```python
from build123d import *

# Parameters (mm, degrees)
ESQUISSE1_W              = 200
ESQUISSE1_H              = 140
BOSS_EXTRU_1_DEPTH       = 6
ESQUISSE8_W              = 31
ESQUISSE8_H              = 60
ESQUISSE8_W_2            = 10
ENL_V_MAT_EXTRU_2_DEPTH  = 6
ESQUISSE9_W              = 20
ESQUISSE9_H              = 6
ENL_V_MAT_EXTRU_3_DEPTH  = 6
ESQUISSE10_W             = 6
ESQUISSE10_H             = 20
ENL_V_MAT_EXTRU_4_DEPTH  = 6
ESQUISSE14_W             = 30
ESQUISSE14_H             = 6
ENL_V_MAT_EXTRU_7_DEPTH  = 6
ESQUISSE15_R             = 10.5
ENL_V_MAT_EXTRU_8_DEPTH  = 6
ESQUISSE19_R             = 2
ENL_V_MAT_EXTRU_11_DEPTH = 245.204832057
ESQUISSE20_R             = 1.5
ENL_V_MAT_EXTRU_12_DEPTH = 245.204832057
ESQUISSE21_R             = 1.5
ESQUISSE21_W             = 20
ESQUISSE21_H             = 6
ENL_V_MAT_EXTRU_13_DEPTH = 10
ESQUISSE23_R             = 1.65
ENL_V_MAT_EXTRU_15_DEPTH = 6
ESQUISSE16_R             = 1.5
ENL_V_MAT_EXTRU_9_DEPTH  = 6
ESQUISSE28_W             = 6
ESQUISSE28_H             = 20
ENL_V_MAT_EXTRU_17_DEPTH = 245.204832057
ESQUISSE29_R             = 1.5
ENL_V_MAT_EXTRU_18_DEPTH = 245.204832057
ESQUISSE35_R             = 1.5
ENL_V_MAT_EXTRU_21_DEPTH = 6
CONG_1_R                 = 1


with BuildPart() as part:
    # Esquisse1 → Boss.-Extru.1 (new body)
    with BuildSketch(Plane.XY):
        with Locations((100, -70)):
            Rectangle(ESQUISSE1_W, ESQUISSE1_H)
    extrude(amount=BOSS_EXTRU_1_DEPTH)

    # Esquisse8 → Enl_v. mat.-Extru.2 (cut)
    with BuildSketch(Plane(origin=(0, 0, 0), x_dir=(-1, 0, 0), z_dir=(0, 0, -1))):
        with Locations((-146, -42)):
            Rectangle(ESQUISSE8_W, ESQUISSE8_H)
        with Locations((-186, -42)):
            Rectangle(ESQUISSE8_W_2, ESQUISSE8_H)
        with Locations((-14, -42)):
            Rectangle(ESQUISSE8_W_2, ESQUISSE8_H)
        with Locations((-54, -42)):
            Rectangle(ESQUISSE8_W, ESQUISSE8_H)
    extrude(amount=-ENL_V_MAT_EXTRU_2_DEPTH, mode=Mode.SUBTRACT)

    # Esquisse9 → Enl_v. mat.-Extru.3 (cut)
    with BuildSketch(Plane(origin=(0, 0, 0), x_dir=(-1, 0, 0), z_dir=(0, 0, -1))):
        with Locations((-150, -3)):
            Rectangle(ESQUISSE9_W, ESQUISSE9_H)
        with Locations((-50, -3)):
            Rectangle(ESQUISSE9_W, ESQUISSE9_H)
    extrude(amount=-ENL_V_MAT_EXTRU_3_DEPTH, mode=Mode.SUBTRACT)

    # Esquisse10 → Enl_v. mat.-Extru.4 (cut)
    with BuildSketch(Plane(origin=(0, 0, 0), x_dir=(-1, 0, 0), z_dir=(0, 0, -1))):
        with Locations((-197, -100)):
            Rectangle(ESQUISSE10_W, ESQUISSE10_H)
        with Locations((-3, -100)):
            Rectangle(ESQUISSE10_W, ESQUISSE10_H)
    extrude(amount=-ENL_V_MAT_EXTRU_4_DEPTH, mode=Mode.SUBTRACT)

    # Esquisse14 → Enl_v. mat.-Extru.7 (cut)
    with BuildSketch(Plane.XY.offset(6)):
        with Locations((100, -25)):
            Rectangle(ESQUISSE14_W, ESQUISSE14_H)
    extrude(amount=-ENL_V_MAT_EXTRU_7_DEPTH, mode=Mode.SUBTRACT)

    # Esquisse15 → Enl_v. mat.-Extru.8 (cut)
    with BuildSketch(Plane.XY.offset(6)):
        with Locations((195, -135)):
            Circle(ESQUISSE15_R)
        with Locations((5, -135)):
            Circle(ESQUISSE15_R)
    extrude(amount=-ENL_V_MAT_EXTRU_8_DEPTH, mode=Mode.SUBTRACT)

    # Esquisse19 → Enl_v. mat.-Extru.11 (cut, through all)
    with BuildSketch(Plane(origin=(0, 0, 0), x_dir=(-1, 0, 0), z_dir=(0, 0, -1))):
        with Locations((-28.75, -67)):
            Circle(ESQUISSE19_R)
        with Locations((-28.75, -17)):
            Circle(ESQUISSE19_R)
        with Locations(Location((-171.25, -17, 0), (0, 0, 180))):
            Circle(ESQUISSE19_R)
        with Locations(Location((-171.25, -67, 0), (0, 0, 180))):
            Circle(ESQUISSE19_R)
    extrude(amount=-ENL_V_MAT_EXTRU_11_DEPTH, mode=Mode.SUBTRACT)

    # Esquisse20 → Enl_v. mat.-Extru.12 (cut, through all)
    with BuildSketch(Plane.XY.offset(6)):
        with Locations((19.495689014, -120.504310986)):
            Circle(ESQUISSE20_R)
        with Locations((19.212846302, -105.506977889)):
            Circle(ESQUISSE20_R)
        with Locations(Location((180.787153698, -105.506977889, 0), (0, 0, 180))):
            Circle(ESQUISSE20_R)
        with Locations((30, -117.5)):
            Circle(ESQUISSE20_R)
        with Locations((30, -92.5)):
            Circle(ESQUISSE20_R)
        with Locations(Location((180.504310986, -120.504310986, 0), (0, 0, 180))):
            Circle(ESQUISSE20_R)
        with Locations(Location((170, -92.5, 0), (0, 0, 180))):
            Circle(ESQUISSE20_R)
        with Locations(Location((170, -117.5, 0), (0, 0, 180))):
            Circle(ESQUISSE20_R)
        with Locations((76.5, -25)):
            Circle(ESQUISSE20_R)
        with Locations((123.5, -25)):
            Circle(ESQUISSE20_R)
    extrude(amount=-ENL_V_MAT_EXTRU_12_DEPTH, mode=Mode.SUBTRACT)

    # Esquisse21 → Enl_v. mat.-Extru.13 (cut)
    with BuildSketch(Plane(origin=(0, 0, 0), x_dir=(-1, 0, 0), z_dir=(0, 0, -1))):
        with Locations((-85, -71)):
            Circle(ESQUISSE21_R)
        with Locations((-115, -71)):
            Circle(ESQUISSE21_R)
        with Locations((-100, -71)):
            Rectangle(ESQUISSE21_W, ESQUISSE21_H)
    extrude(amount=-ENL_V_MAT_EXTRU_13_DEPTH, mode=Mode.SUBTRACT)

    # Esquisse23 → Enl_v. mat.-Extru.15 (cut)
    with BuildSketch(Plane(origin=(0, 0, 0), x_dir=(-1, 0, 0), z_dir=(0, 0, -1))):
        with Locations(Location((-4.2, -3.5, 0), (0, 0, 180))):
            Circle(ESQUISSE23_R)
        with Locations((-195.8, -3.5)):
            Circle(ESQUISSE23_R)
    extrude(amount=-ENL_V_MAT_EXTRU_15_DEPTH, mode=Mode.SUBTRACT)

    # Esquisse16 → Enl_v. mat.-Extru.9 (cut)
    with BuildSketch(Plane(origin=(0, 0, 0), x_dir=(-1, 0, 0), z_dir=(0, 0, -1))):
        with Locations((-3, -83)):
            Circle(ESQUISSE16_R)
        with Locations(Location((-197, -117, 0), (0, 0, 180))):
            Circle(ESQUISSE16_R)
        with Locations((-197, -83)):
            Circle(ESQUISSE16_R)
        with Locations((-3, -117)):
            Circle(ESQUISSE16_R)
    extrude(amount=-ENL_V_MAT_EXTRU_9_DEPTH, mode=Mode.SUBTRACT)

    # Esquisse28 → Enl_v. mat.-Extru.17 (cut, through all)
    with BuildSketch(Plane.XY.offset(6)):
        with Locations((3, -42)):
            Rectangle(ESQUISSE28_W, ESQUISSE28_H)
        with Locations((197, -42)):
            Rectangle(ESQUISSE28_W, ESQUISSE28_H)
    extrude(amount=-ENL_V_MAT_EXTRU_17_DEPTH, mode=Mode.SUBTRACT)

    # Esquisse29 → Enl_v. mat.-Extru.18 (cut, through all)
    with BuildSketch(Plane(origin=(0, 0, 0), x_dir=(-1, 0, 0), z_dir=(0, 0, -1))):
        with Locations((-197, -25)):
            Circle(ESQUISSE29_R)
        with Locations((-197, -59)):
            Circle(ESQUISSE29_R)
        with Locations(Location((-3, -59, 0), (0, 0, 180))):
            Circle(ESQUISSE29_R)
        with Locations(Location((-3, -25, 0), (0, 0, 180))):
            Circle(ESQUISSE29_R)
    extrude(amount=-ENL_V_MAT_EXTRU_18_DEPTH, mode=Mode.SUBTRACT)

    # Esquisse35 → Enl_v. mat.-Extru.21 (cut)
    with BuildSketch(Plane(origin=(0, 0, 0), x_dir=(-1, 0, 0), z_dir=(0, 0, -1))):
        with Locations((-167, -3)):
            Circle(ESQUISSE35_R)
        with Locations((-131.260401336, -3)):
            Circle(ESQUISSE35_R)
        with Locations((-100, -3)):
            Circle(ESQUISSE35_R)
        with Locations((-67, -3)):
            Circle(ESQUISSE35_R)
        with Locations((-33, -3)):
            Circle(ESQUISSE35_R)
    extrude(amount=-ENL_V_MAT_EXTRU_21_DEPTH, mode=Mode.SUBTRACT)

    # Cong_1
    cong_1_edges = [part.edges().sort_by_distance(p)[0] for p in [
        (200, -110, 3),
        (200, -90, 3),
        (0, -90, 3),
        (0, -110, 3),
        (185.766907344, -140, 3),
        (200, -125.766907344, 3),
        (14.233092656, -140, 3),
        (0, -125.766907344, 3),
        (0, -52, 3),
        (0, -32, 3),
        (200, -32, 3),
        (200, -52, 3),
        (0, 0, 3),
        (200, 0, 3),
        (160, 0, 3),
        (140, 0, 3),
        (60, 0, 3),
        (40, 0, 3),
    ]]
    fillet(cong_1_edges, radius=CONG_1_R)


solid = part.part
```
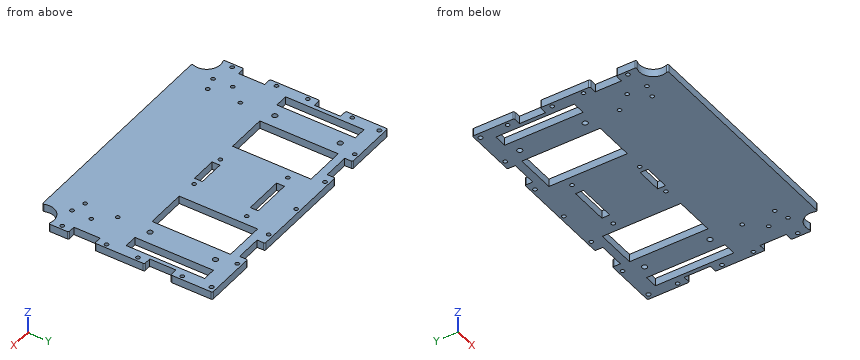
Input: part model. Units: mm. Frame: model coordinates. Coordinates: 2 decimals unless noted, no trailing zeros. Write each loop counter-clockwise with the first axis right and the second up, starting at its lowest first coordinate (ties: lowest second). Pieces come first, ordered by that corner, then holes. Notation, with made-up numbers: (7.5, 86) - (33.5, 86) arc R6 cw to (33.5, 96) - close; hole circle Ø1 at (-0.5, 8). An arc over 180 degrees is marked (long way). Put each result on its own line as item: value. Start each with the question number.
1) Contact query for flat-ended pins moving along their axis: pin 1 (1.8 mm diameter, centred on x = 3, y = -59, fed in from -Z); pin 2 (1.8 mm diameter, centred on x = 149.5, z = 1.5, fed in from +Y). Output: stop coordinate, or through.
2) Cut plane A-A (x = 43). Return the cut outline in (y, z), plus the area to 3 significant figures.
3) Cut plane C-C (y = -100.5). Return the cut outline in (x, z).
4) Cut plane B-B (z = 1.45). State how many separate pieces and enclosed holes the cut face has, plus the area to 3 significant figures.
5) Ray query, L1, parallel to X at y = -46.5, z = 2; L2, parallel to X at y = -27, z = 1.7; L3, parallel to Y at x = 91.5, z = 0.85. Return the intervals inside material, ascending.
Resolved:
1. pin 1: passes through
1. pin 2: stops at y = -6
2. outline: (-140, 0) - (-72, 0) - (-72, 6) - (-140, 6) - close; (-12, 0) - (-6, 0) - (-6, 6) - (-12, 6) - close
2. area: 444 mm2
3. outline: (6, 0) - (194, 0) - (194, 6) - (6, 6) - close
4. separate pieces: 1
4. enclosed holes: 37
4. area: 21,400 mm2
5. L1: x = 6 to 9, 19 to 38.5, 69.5 to 130.5, 161.5 to 181, 191 to 194
5. L2: x = 0 to 9, 19 to 38.5, 69.5 to 85, 115 to 130.5, 161.5 to 181, 191 to 200
5. L3: y = -140 to -74, -68 to -28, -22 to 0
